Design review of the part built by this model. Coordinates are the model's own, in mm. A direction names the side the tool comes from. Coordinates: 2 decimals unless noted, no trailing zeros. Order: outer loops, then holes, each group sorted by start corner. A loop starts at its lowest first (then second) coordinate and runs counter-clockwise, first axis right, second up. Notation, with made-up numbers: (29, 18) - (41, 18) arc R23 ccw to (41, 32) - close; hole circle Ø8 at (75, -11). An arc over 180 degrees is marked (long way). Write each question's results on one line, items separated by ' | '. Start each with the question number.
```python
from build123d import *

# Parameters (mm, degrees)
BOSS_EXTRUDE1_START = 15
BOSS_EXTRUDE1_DEPTH = 279.5
SKETCH3_W           = 107
SKETCH3_H           = 93.25
CUT_EXTRUDE1_DEPTH  = 173.25
SKETCH4_R           = 20.5
CUT_EXTRUDE2_DEPTH  = 304.90560212
CUT_EXTRUDE3_START  = -50
CUT_EXTRUDE3_DEPTH  = 50
SKETCH7_R           = 2.3
CUT_EXTRUDE5_DEPTH  = 305.779129174
CUT_EXTRUDE8_START  = -304.43404156
SKETCH11_R          = 3.8
CUT_EXTRUDE8_DEPTH  = 311.43404156
SKETCH14_R          = 1.93
CUT_EXTRUDE9_DEPTH  = 7.25
SKETCH18_W          = 44.336356413
SKETCH18_H          = 6
CUT_EXTRUDE10_DEPTH = 125.5
CUT_EXTRUDE12_DEPTH = 100.5
SKETCH20_W          = 88.672712826
SKETCH20_H          = 6
BOSS_EXTRUDE2_DEPTH = 75.5
SCREW_HEAD_HOLE_R   = 3.3
SCREW_HEAD_HOLE_R_2 = 1.45
CUT_EXTRUDE13_DEPTH = 7


with BuildPart() as part:
    # Sketch1 → Boss-Extrude1 (new body)
    with BuildSketch(Plane.XY.offset(BOSS_EXTRUDE1_START)):
        with BuildLine():
            Line((-69.190786959, -30.525), (-35, -30.525))
            Line((-35, -30.525), (-35, -46.625))
            Line((-35, -46.625), (35, -46.625))
            Line((35, -46.625), (35, -30.525))
            Line((35, -30.525), (69.190786959, -30.525))
            ThreePointArc((69.190786959, -30.525), (0, -75.625), (-69.190786959, -30.525))
        make_face()
    extrude(amount=BOSS_EXTRUDE1_DEPTH)

    # Sketch3 → Cut-Extrude1 (cut)
    with BuildSketch(Plane(origin=(0, 0, 15), x_dir=(-1, 0, 0), z_dir=(0, 0, -1))):
        Rectangle(SKETCH3_W, SKETCH3_H)
    extrude(amount=-CUT_EXTRUDE1_DEPTH, mode=Mode.SUBTRACT)

    # Sketch4 → Cut-Extrude2 (cut, through all)
    with BuildSketch(Plane(origin=(0, -46.625, 0), x_dir=(1, 0, 0), z_dir=(0, 1, 0))):
        with Locations(Location((0, -269.5, 0), (0, 0, 270))):
            Circle(SKETCH4_R)
    extrude(amount=-CUT_EXTRUDE2_DEPTH, mode=Mode.SUBTRACT)

    # Sketch2 → Cut-Extrude3 (cut)
    with BuildSketch(Plane.XY.offset(294.5).offset(CUT_EXTRUDE3_START)):
        with BuildLine():
            Line((-35, -30.525), (-35, -38.575))
            Line((-35, -38.575), (-65.04698302, -38.575))
            ThreePointArc((-65.04698302, -38.575), (-67.239462723, -34.612068383), (-69.190786959, -30.525))
            Line((-69.190786959, -30.525), (-35, -30.525))
        make_face()
    cut_extrude3 = extrude(amount=CUT_EXTRUDE3_DEPTH, mode=Mode.SUBTRACT)

    # Mirror1: Cut-Extrude3 across plane
    add(cut_extrude3.mirror(Plane(origin=(0, 0, 0), x_dir=(0, 0, 1), z_dir=(1, 0, 0))), mode=Mode.SUBTRACT)

    # Sketch7 → Cut-Extrude5 (cut, through all)
    with BuildSketch(Plane(origin=(0, -38.575, 0), x_dir=(1, 0, 0), z_dir=(0, 1, 0))):
        with Locations(Location((45, -257, 0), (0, 0, 180))):
            Circle(SKETCH7_R)
        with Locations(Location((45, -282, 0), (0, 0, 180))):
            Circle(SKETCH7_R)
    cut_extrude5 = extrude(amount=-CUT_EXTRUDE5_DEPTH, mode=Mode.SUBTRACT)

    # Mirror2: Cut-Extrude5 across plane
    add(cut_extrude5.mirror(Plane(origin=(0, 0, 0), x_dir=(0, 0, 1), z_dir=(1, 0, 0))), mode=Mode.SUBTRACT)

    # Sketch11 → Cut-Extrude8 (cut)
    with BuildSketch(Plane(origin=(0, -52.075, 0), x_dir=(1, 0, 0), z_dir=(0, 1, 0)).offset(CUT_EXTRUDE8_START)):
        with Locations(Location((45, -282, 0), (0, 0, 180))):
            Circle(SKETCH11_R)
        with Locations(Location((45, -257, 0), (0, 0, 180))):
            Circle(SKETCH11_R)
    cut_extrude8 = extrude(amount=CUT_EXTRUDE8_DEPTH, mode=Mode.SUBTRACT)

    # Mirror3: Cut-Extrude8 across plane
    add(cut_extrude8.mirror(Plane(origin=(0, 0, 0), x_dir=(0, 0, 1), z_dir=(1, 0, 0))), mode=Mode.SUBTRACT)

    # Sketch14 → Cut-Extrude9 (cut)
    with BuildSketch(Plane(origin=(0, -30.525, 0), x_dir=(1, 0, 0), z_dir=(0, 1, 0))):
        with Locations(Location((62.5, -27.45, 0), (0, 0, 180))):
            Circle(SKETCH14_R)
        with Locations(Location((62.5, -82.35, 0), (0, 0, 180))):
            Circle(SKETCH14_R)
    cut_extrude9 = extrude(amount=-CUT_EXTRUDE9_DEPTH, mode=Mode.SUBTRACT)

    # Mirror4: Cut-Extrude9 across plane
    add(cut_extrude9.mirror(Plane(origin=(0, 0, 0), x_dir=(0, 0, 1), z_dir=(1, 0, 0))), mode=Mode.SUBTRACT)

    # Sketch18 → Cut-Extrude10 (cut)
    with BuildSketch(Plane(origin=(0, 0, 15), x_dir=(-1, 0, 0), z_dir=(0, 0, -1))):
        with Locations((-22.168178207, -53.125)):
            Rectangle(SKETCH18_W, SKETCH18_H)
        with Locations((22.168178207, -53.125)):
            Rectangle(SKETCH18_W, SKETCH18_H)
        with BuildLine():
            Line((42.207819181, -56.625), (0, -56.625))
            Line((0, -56.625), (0, -64.625))
            Line((0, -64.625), (28.486839066, -64.625))
            ThreePointArc((28.486839066, -64.625), (35.572934602, -61.011941035), (42.207819181, -56.625))
        make_face()
        with BuildLine():
            Line((0, -64.625), (0, -56.625))
            Line((0, -56.625), (-42.207819181, -56.625))
            ThreePointArc((-42.207819181, -56.625), (-35.572934602, -61.011941035), (-28.486839066, -64.625))
            Line((-28.486839066, -64.625), (0, -64.625))
        make_face()
        with BuildLine():
            Line((42.207819181, -56.625), (0, -56.625))
            Line((0, -56.625), (0, -64.625))
            Line((0, -64.625), (28.486839066, -64.625))
            ThreePointArc((28.486839066, -64.625), (35.572934602, -61.011941035), (42.207819181, -56.625))
        make_face()
        with BuildLine():
            Line((0, -64.625), (0, -56.625))
            Line((0, -56.625), (-42.207819181, -56.625))
            ThreePointArc((-42.207819181, -56.625), (-35.572934602, -61.011941035), (-28.486839066, -64.625))
            Line((-28.486839066, -64.625), (0, -64.625))
        make_face()
        with BuildLine():
            Line((-42.207819181, -56.625), (0, -56.625))
            Line((0, -56.625), (0, -56.125))
            Line((0, -56.125), (-44.336356413, -56.125))
            ThreePointArc((-44.336356413, -56.125), (-37.468701056, -60.779511824), (-30.117416058, -64.625))
            Line((-30.117416058, -64.625), (-28.486839066, -64.625))
            ThreePointArc((-28.486839066, -64.625), (-35.572934602, -61.011941035), (-42.207819181, -56.625))
        make_face()
        with BuildLine():
            Line((0, -56.125), (0, -56.625))
            Line((0, -56.625), (42.207819181, -56.625))
            ThreePointArc((42.207819181, -56.625), (35.572934602, -61.011941035), (28.486839066, -64.625))
            Line((28.486839066, -64.625), (30.117416058, -64.625))
            ThreePointArc((30.117416058, -64.625), (37.468701056, -60.779511824), (44.336356413, -56.125))
            Line((44.336356413, -56.125), (0, -56.125))
        make_face()
        with BuildLine():
            Line((-42.207819181, -56.625), (0, -56.625))
            Line((0, -56.625), (0, -56.125))
            Line((0, -56.125), (-44.336356413, -56.125))
            ThreePointArc((-44.336356413, -56.125), (-37.468701056, -60.779511824), (-30.117416058, -64.625))
            Line((-30.117416058, -64.625), (-28.486839066, -64.625))
            ThreePointArc((-28.486839066, -64.625), (-35.572934602, -61.011941035), (-42.207819181, -56.625))
        make_face()
        with BuildLine():
            Line((0, -56.125), (0, -56.625))
            Line((0, -56.625), (42.207819181, -56.625))
            ThreePointArc((42.207819181, -56.625), (35.572934602, -61.011941035), (28.486839066, -64.625))
            Line((28.486839066, -64.625), (30.117416058, -64.625))
            ThreePointArc((30.117416058, -64.625), (37.468701056, -60.779511824), (44.336356413, -56.125))
            Line((44.336356413, -56.125), (0, -56.125))
        make_face()
    extrude(amount=-CUT_EXTRUDE10_DEPTH, mode=Mode.SUBTRACT)

    # Sketch19 → Cut-Extrude12 (cut)
    with BuildSketch(Plane(origin=(0, 0, 40), x_dir=(-1, 0, 0), z_dir=(0, 0, -1))):
        with BuildLine():
            ThreePointArc((-30.117416058, -64.625), (0, -71.125), (30.117416058, -64.625))
            Line((30.117416058, -64.625), (-30.117416058, -64.625))
        make_face()
    extrude(amount=-CUT_EXTRUDE12_DEPTH, mode=Mode.SUBTRACT)

    # Sketch20 → Boss-Extrude2 (add)
    with BuildSketch(Plane(origin=(0, 0, 65), x_dir=(-1, 0, 0), z_dir=(0, 0, -1))):
        with Locations((0, -53.125)):
            Rectangle(SKETCH20_W, SKETCH20_H)
    extrude(amount=-BOSS_EXTRUDE2_DEPTH)

    # screw head hole → Cut-Extrude13 (cut)
    # profile 1 of 2: a face of its own
    with BuildSketch(Plane(origin=(0, 0, 15), x_dir=(-1, 0, 0), z_dir=(0, 0, -1))):
        with Locations((0, -68.825)):
            Circle(SCREW_HEAD_HOLE_R)
        with Locations((0, -68.825)):
            Circle(SCREW_HEAD_HOLE_R_2, mode=Mode.SUBTRACT)
    # profile 2 of 2: a face of its own
    with BuildSketch(Plane(origin=(0, 0, 15), x_dir=(-1, 0, 0), z_dir=(0, 0, -1))):
        with Locations((0, -68.825)):
            Circle(SCREW_HEAD_HOLE_R_2)
    extrude(amount=-CUT_EXTRUDE13_DEPTH, mode=Mode.SUBTRACT)


solid = part.part
```
(1) Take a section at C-C (z = 269.5). State the section outline as (x, y) points (3 decimals).
(2) Tool access review of faces 1 (the face through (-35, -40, 229)), 2 (the face through (-44.336, -53, 40)), 3 (the face through (0, -67, 40)), 4 (the face through (44, -38, 188.25)), 5 (the face through (43, -45.075, 280)): name each direction out of +Z, -Z, +X, -X, +Y, -Y from which nothing blocks a thin tool from reaching the whole face with its end or side.
(3) Take a section at D-D (z = 239). State the section outline as (x, y) points (3 decimals).
(4) Clearance check with flat-ended pins moving along their axes: pin 1 (6 mm diameter, centred on x = 43.5, z = 255.5, fed in from -Y); pin 2 (6 mm diameter, centred on x = 62.5, z = 27.45, fed in from -Y); pin 3 (8 mm diameter, centred on x = 43.5, z = 85, fed in from -Y); pin 4 (3 mm diameter, centred on x = -45, z = 257, fed in from +Y). State where each tip first meets the part, or that it passes through.
(5) To check wall thickness, follow line 1 along Z through (x, y) = (-62.5, -33.5); line 2 along Z through (x, y) = (-45, -42); line 3 along X through (y, z) = (-41.75, 282). State the ranges of each line that lie inside material, in increasing order. Write a range as [from, to].
(6) Mouldability with a two-part tool opening along Y and no side actions: class faces 6 (the face through (53.5, -39, 100)), 7 (the face through (1, -62, 140.5)), 8 (the face through (1, -46.625, 122)) as +Y half, -Y half, draft (parallel to the pull), parting line (faces both ways), or undercut.
(7) Take a section at B-B (x = -15). State the section outline as (y, z) points (3 decimals).
Worked out:
1) outline: (-65.047, -38.575) arc R75.625 ccw to (-20.5, -72.793) - (-20.5, -46.625) - (-35, -46.625) - (-35, -38.575) - close; (20.5, -72.793) arc R75.625 ccw to (65.047, -38.575) - (35, -38.575) - (35, -46.625) - (20.5, -46.625) - close
2) face 1: +Z, -Z, +Y | face 2: -Z | face 3: none | face 4: -Z, +Y | face 5: -Y
3) outline: (-69.191, -30.525) arc R75.625 ccw to (69.191, -30.525) - (35, -30.525) - (35, -46.625) - (-35, -46.625) - (-35, -30.525) - close
4) pin 1: y = -63.87 | pin 2: y = -46.68 | pin 3: y = -64.49 | pin 4: through
5) line 1: [15, 25.52], [29.38, 80.42], [84.28, 244.5] | line 2: [188.25, 254.7], [259.3, 279.7], [284.3, 294.5] | line 3: [-63.06, -47.3], [-42.7, -35], [35, 42.7], [47.3, 63.06]
6) face 6: draft | face 7: undercut | face 8: +Y half
7) outline: (-74.122, 15) - (-64.625, 15) - (-64.625, 40) - (-69.568, 40) - (-69.568, 140.5) - (-56.125, 140.5) - (-56.125, 65) - (-50.125, 65) - (-50.125, 15) - (-46.625, 15) - (-46.625, 255.527) - (-74.122, 255.527) - close; (-74.122, 283.473) - (-46.625, 283.473) - (-46.625, 294.5) - (-74.122, 294.5) - close
